Input: part model. Units: mm. Frame: model coordinates. Coordinates: 2 decimals unless noted, no trailing zeros. Order: outer loops, then holes, each group sorted by start corner. A loop starts at its lowest first (then second) coordinate and runs counter-clockwise, first axis right, second up. Notation, with made-up numbers: (71, -14.5) - (115, -14.5) arc R25 ccw to (115, 7.5) - close; hole circle Ø10 at (-15, 70). An arc over 180 degrees is marked (long way). Answer as CSV lines item,"result". Start each with the question number.
Item 1: Section A-A (z = 1.1). Output: boundary loops of the cut face in (x, y), and give its area (3 significant figures).
Item 2: Section C-C (x = -201). Output: boundary loops of the cut face in (y, z).
Item 3: Section B-B (y = -433.5). Output: boundary loops of the cut face in (x, z), and give its area (3 significant figures).
Item 4: Material intervals for line 1 along Y through (x, z) = (-244, 0.95); line 2 along X through (y, z) = (403, 2); line 3 along Y through (x, z) = (-23, 2.05), sorted ascending.
Autodesk Inventor part; units mm, degrees
ref_plane "Work Plane1" through (0, 0, 0) normal (0, 0, 1) x (1, 0, 0)
ref_plane "YZ Plane" through (0, 0, 0) normal (1, 0, 0) x (0, 1, 0)
ref_plane "XZ Plane" through (0, 0, 0) normal (0, 1, 0) x (-1, 0, 0)
ref_plane "Work Plane1" through (0, 0, 0) normal (0, 0, 1) x (1, 0, 0)
sketch "Sketch1" plane through (0, 0, 0) normal (0, 0, 1) x (1, 0, 0)
  line L0 (500, -288.6751) -> (0, -577.3503)
  line L1 (0, -577.3503) -> (-500, -288.6751)
  line L2 (-500, -288.6751) -> (-500, 288.6751)
  line L3 (-500, 288.6751) -> (0, 577.3503)
  line L4 (0, 577.3503) -> (500, 288.6751)
  line L5 (500, 288.6751) -> (500, -288.6751)
  point P0 (0, 0)
  point P1 (0, 0)
  point P2 (0, 0)
  dimension "d1" = 500
extrude "Extrusion1" add sketch "Sketch1" along normal blind 4
properties part number "Top" material "Glass"
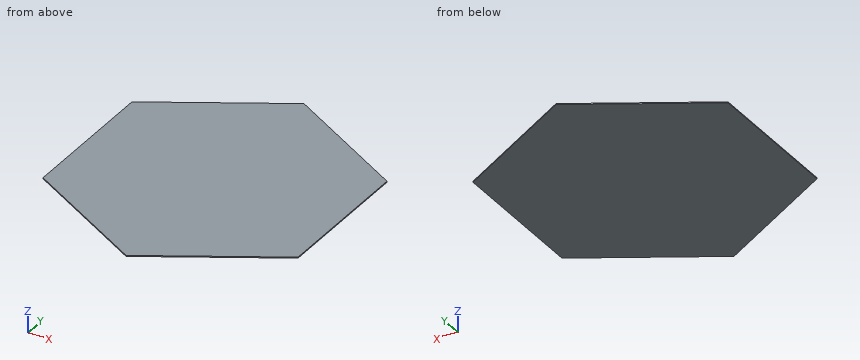
Determined:
1,outline,"(-500, -288.68) - (0, -577.35) - (500, -288.68) - (500, 288.68) - (0, 577.35) - (-500, 288.68) - close"
1,area,"866,000 mm^2"
2,outline,"(-461.3, 0) - (461.3, 0) - (461.3, 4) - (-461.3, 4) - close"
3,outline,"(-249.16, 0) - (249.16, 0) - (249.16, 4) - (-249.16, 4) - close"
3,area,"1,990 mm^2"
4,line 1,"y = -436.48 to 436.48"
4,line 2,"x = -301.98 to 301.98"
4,line 3,"y = -564.07 to 564.07"
